Here's how the part is built. I have some questions about the finished solid (model axes, mm). A direction names the side the tool comes from. Round coordinates to 2 decimals unless told otherwise and drop trailing zeros. Write each loop counter-clockwise with the first axis right and the second up, starting at its lowest first coordinate (ties: lowest second). Pieces come first, ordered by that corner, then holes. Notation, with made-up numbers: M -26.5,55.5 L -11.5,55.5 A27 ccw -11.5,88.5 Z; hole C 12.25,48 d2. An arc over 180 degrees is marked long. Use one line per item in the form item = value. Start each with the question number.
Q1. For faces 1 (the face through (-131.5, -19, 62)), 2 (the face through (-68, -18, 125)), which set-ups out of +Z, -Z, +X, -X, +Y, -Y let a thin tool reach every point of the face, with its end or its side?
Q2. I want a section at D-D on x = -116. List the corners of the cut face in (y, z) for me.
Q3. I want a section at B-B on z = 35.5. List the corners of the cut face in (x, y) for me.
Q4. I need wall thicknesses on line 1 along X through (y, z) = (-29, 123); line 2 along Z through (x, y) = (-30, -33); line 3 along X through (y, z) = (-28, 85). Which ranges of each line are inside material? Lowest first, please. Write a range as from..to.
Q5. We'd pull the mould along X, two halves only. Please class faces 3 (the face through (-18, -11.5, 112)), 4 (the face through (-135, -18, 62)), 5 (the face through (-67, -1, 63)): +X half, -X half, draft (parallel to the pull), parting line (faces both ways), or undercut.
Q6. I'm going to push flat-ended pins straight in: pin 1 Ø3.5 at (x, z) = (-17, 111.5) entering from -Y; pin 2 Ø1.8 at (x, z) = (-30, 1.75) entering from -Y; pin 3 Ø1.5 at (x, z) = (-100, 106.5) entering from -Y. Where does each tip first touch, or does it pass through?
Q7. I want a section at C-C on x = -12.7. List the corners of the cut face in (y, z) for me.
Q8. I want a section at A-A on y = -9.5. List the corners of the cut face in (x, z) for me.
```python
from build123d import *

# Parameters (mm, degrees)
F0_W      = 135
F0_H      = 125
F1_DEPTH  = 35
F2_T      = -3.5
F3_R      = 1.45
F3_R_2    = 1.55
F4_DEPTH  = 8
F5_R      = 1
F6_DEPTH  = 8
F7_W      = 135
F7_H      = 125
F8_DEPTH  = 1
F9_R      = 1.830023
F10_DEPTH = 5
F11_R     = 2.785388
F12_DEPTH = 5


with BuildPart() as f1:
    # F0 (on Front) → F1 (new body)
    with BuildSketch(Plane.XZ):
        with Locations((-67.5, 62.5)):
            Rectangle(F0_W, F0_H)
    extrude(amount=F1_DEPTH)

    # F2
    f2_openings = [f1.faces().sort_by_distance(p)[0] for p in [
        (-67.5, -35, 62.5),
    ]]
    offset(amount=F2_T, openings=f2_openings)

    # F3 (on face) → F4 (join)
    with BuildSketch(Plane.XZ.offset(3.5)):
        with Locations((-99.5, 106.5)):
            Circle(F3_R)
        with Locations((-99.5, 31.5)):
            Circle(F3_R)
        with Locations((-45.4, 111.5)):
            Circle(F3_R_2)
        with Locations((-17.5, 111.5)):
            Circle(F3_R_2)
        with Locations((-12.7, 59.6)):
            Circle(F3_R_2)
        with Locations((-60.6, 60.7)):
            Circle(F3_R_2)
    extrude(amount=F4_DEPTH)

    # F5 (on face) → F6 (cut)
    with BuildSketch(Plane.XZ.offset(35)):
        with Locations((-30, 123.25)):
            Circle(F5_R)
        with Locations((-1.75, 85)):
            Circle(F5_R)
        with Locations((-30, 1.75)):
            Circle(F5_R)
        with Locations((-105, 1.75)):
            Circle(F5_R)
        with Locations((-133.25, 40)):
            Circle(F5_R)
        with Locations((-105, 123.25)):
            Circle(F5_R)
    extrude(amount=-F6_DEPTH, mode=Mode.SUBTRACT)

    # F7 (on face) → F8 (cut)
    with BuildSketch(Plane(origin=(0, 0, 0), x_dir=(-1, 0, 0), z_dir=(0, 1, 0))):
        with Locations((67.5, 62.5)):
            Rectangle(F7_W, F7_H)
    extrude(amount=-F8_DEPTH, mode=Mode.SUBTRACT)

    # F9 (on face) → F10 (cut)
    with BuildSketch(Plane.XZ.offset(11.5)):
        with Locations((-99.5, 106.5)):
            Circle(F9_R)
    extrude(amount=-F10_DEPTH, mode=Mode.SUBTRACT)

    # F11 (on face) → F12 (cut)
    with BuildSketch(Plane.XZ.offset(11.5)):
        with Locations((-99.5, 31.5)):
            Circle(F11_R)
    extrude(amount=-F12_DEPTH, mode=Mode.SUBTRACT)


solid = f1.part
```
Reported:
q1.face_1 = -Y
q1.face_2 = +Z, +X, -X, +Y, -Y
q2.outline = M -35,0 L -1,0 L -1,125 L -35,125 L -35,121.5 L -3.5,121.5 L -3.5,3.5 L -35,3.5 Z
q3.outline = M -135,-35 L -131.5,-35 L -131.5,-3.5 L -3.5,-3.5 L -3.5,-35 L 0,-35 L 0,-1 L -135,-1 Z
q4.line_1 = -135..-105.97, -104.03..-30.97, -29.03..0
q4.line_2 = 0..0.75, 2.75..3.5, 121.5..122.25, 124.25..125
q4.line_3 = -135..-131.5, -3.5..-2.75, -0.75..0
q5.face_3 = undercut
q5.face_4 = -X half
q5.face_5 = draft
q6.pin_1 = -11.5
q6.pin_2 = -27
q6.pin_3 = -6.5
q7.outline = M -35,0 L -1,0 L -1,125 L -35,125 L -35,121.5 L -3.5,121.5 L -3.5,61.15 L -11.5,61.15 L -11.5,58.05 L -3.5,58.05 L -3.5,3.5 L -35,3.5 Z
q8.outline = M -135,0 L 0,0 L 0,125 L -135,125 Z; C -60.6,60.7 d3.1; C -45.4,111.5 d3.1; C -17.5,111.5 d3.1; C -12.7,59.6 d3.1; hole M -131.5,3.5 L -3.5,3.5 L -3.5,121.5 L -131.5,121.5 Z
